Autodesk Inventor part; units mm, degrees
ref_plane "YZ Plane" through (0, 0, 0) normal (1, 0, 0) x (0, 1, 0)
ref_plane "XZ Plane" through (0, 0, 0) normal (0, 1, 0) x (-1, 0, 0)
ref_plane "XY Plane" through (0, 0, 0) normal (0, 0, 1) x (1, 0, 0)
sketch "Sketch1" plane through (0, 0, 0) normal (0, 0, 1) x (1, 0, 0)
  circle A0 centre (192, 3.5) radius 5.5
  circle A1 centre (-192, 633) radius 5.5
  circle A2 centre (-192, 633) radius 5.5
  arc A3 (-179.1945, 640.8115) -> (-204.8055, 625.1885) centre (-192, 633) ccw
  circle A4 centre (192, 3.5) radius 5.5
  arc A5 (179.1945, -4.3115) -> (204.8055, 11.3115) centre (192, 3.5) ccw
  line L0 (-179.1945, 640.8115) -> (204.8055, 11.3115)
  line L1 (179.1945, -4.3115) -> (-204.8055, 625.1885)
  point P0 (0, 0)
  dimension "d2" = 30
  dimension "d3" = 11
  dimension "d4" = 11
  dimension "d5" = 30
extrude "Extrusion2" add sketch "Sketch1" along normal blind 6
properties part number "90-08-0850" material "Steel, Mild"
Work out the finished part from the listing and answer in its coordinate system (mm). Give positions to 0.01 mm unless a question says otherwise; leave off trailing zeros. Loops run counter-clockwise (first coordinate to the right, second up) from the corner with the lowest first, then second, coordinate; pieces in that order, holes last. Notation, with made-up numbers: (64.5, 32) -> (97.5, 32) arc R4 ccw to (97.5, 39) -> close; hole circle Ø11 at (1.25, -34). An arc over 180 degrees is marked (long way). Use CSV: the item, a comma, the result in double quotes.
1. The part is cut by section C-C (y = 78). Write down the section's boundary in (x, z), then the cut area to 3 significant figures.
Found:
outline,"(128.98, 0) -> (164.12, 0) -> (164.12, 6) -> (128.98, 6) -> close"
area,"211 mm^2"
2. A flat-ended cylindrical pin translates along its axis: pin 1 Ø2 at (y, z) = (497.5, 2.5) entering from -X. Find the tip coordinate at first contact, or state that the pin passes through.
Found:
pin 1,"x = -127.52"
3. The part is cut by section B-B (x = 27). Write down the section's boundary in (y, z), then the cut area to 3 significant figures.
Found:
outline,"(245.18, 0) -> (302.79, 0) -> (302.79, 6) -> (245.18, 6) -> close"
area,"346 mm^2"
4. Straight lines are drawn through the part: line 1 (Y direction, x = 192, z = 4.1); line 2 (Y direction, x = -192, z = 2.4); line 3 (X direction, y = 633, z = 4.1). For each, find the intervals that lie inside material, in ascending order.
Found:
line 1,"-11.5 to -2, 9 to 32.3"
line 2,"604.2 to 627.5, 638.5 to 648"
line 3,"-207 to -197.5, -186.5 to -174.43"
5. The part is cut by section A-A (z = 2.3). Write down the section's boundary in (x, y).
Found:
outline,"(-204.81, 625.19) -> (179.19, -4.31) arc R15 ccw to (204.81, 11.31) -> (-179.19, 640.81) arc R15 ccw to start; hole circle Ø11 at (-192, 633); hole circle Ø11 at (192, 3.5)"
